Build history of the part. All positions in model axes, mm. Face numbers are marked on the shaded views. A direction names the side the tool comes from. Give positions to 0.01 mm unless a question says otherwise; leave off trailing zeros. Loops run counter-clockwise (first coordinate to the right, second up) from the corner with the lowest first, then second, coordinate; pieces in that order, holes last. Notation, with made-up numbers: M 59.5,57.25 L 64.5,57.25 A22 ccw 64.5,92.25 Z; hole C 61.5,-15.5 d8. An arc over 180 degrees is marked long. Answer as a JSON object with one key per item and string values. Group by question number.
1. Drop flat-ended pins along their axis: pin 1 Ø1.5 at (x, y) = (-16, -45.5) entering from +Z; pin 2 Ø4 at (x, z) = (-5, 3.5) entering from -Y; pin 3 Ø8 at (y, z) = (2.5, -1) entering from +X. Give the stop position or say it passes through.
2. Slice it at C-C (z = 12). List the corners of the cut face in (x, y).
3. Slice it at A-A (z = -6). List the corners of the cut face in (x, y).
4. Slice it at D-D (z = 23). List the corners of the cut face in (x, y), then the cut area to 3 significant figures.
5. 3-axis set-ups, long thin cutter, end or side, ignore diameter. For the marked faces 1, 2, 3, 4 and 5: which of +Z, -Z, +X, -X, +Y, -Y reach the whole face in a straight line?
6. Mould opens along X. For the marked faces 6, 7 and 8 say: released by +X, released by -X, zero draft, split by the parting line, or undercut.
7. Drill centre lines: line 1 along Y through (x, z) = (0, -3); line 2 along Z through (x, y) = (2.5, -22.5); line 3 along Z through (x, y) = (3, -60). Where is each one in solid material? Low to high. Write a range as [from, to].
8. Slice it at B-B (x = 0). List the corners of the cut face in (y, z), then the cut area to 3 significant figures.
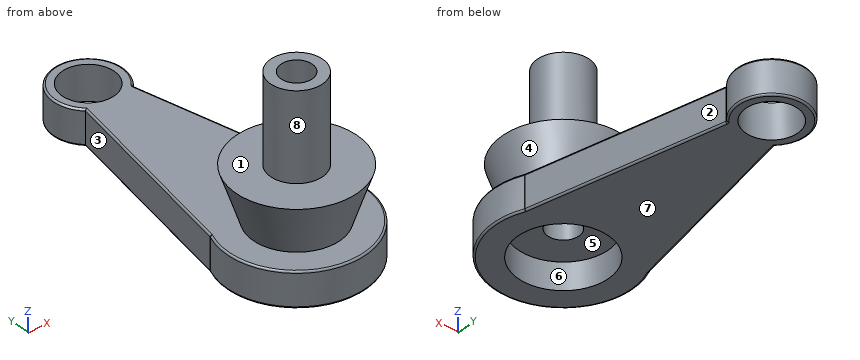
from build123d import *

# Parameters (mm, degrees)
BOSS_EXTRUDE2_DEPTH = 10
SKETCH11_R          = 7.5
CUT_EXTRUDE1_DEPTH  = 11
SKETCH12_R          = 12.5
SKETCH13_R          = 17.5
SKETCH16_R          = 7.5
BOSS_EXTRUDE3_DEPTH = 25
SKETCH17_R          = 13
CUT_EXTRUDE2_DEPTH  = 7.7
FILLET2_R           = 0.5
CUT_EXTRUDE3_REACH  = 44.3
SKETCH18_R          = 4.5


with BuildPart() as part:
    # Sketch10 → Boss-Extrude2 (new body)
    with BuildSketch(Plane.XY):
        with BuildLine():
            Line((-7, 12.658044745), (-18.304628492, -42.341955255))
            ThreePointArc((-18.304628492, -42.341955255), (0, -70.400526826), (18.304628492, -42.341955255))
            Line((18.304628492, -42.341955255), (7, 12.658044745))
            ThreePointArc((7, 12.658044745), (0, 29.799473174), (-7, 12.658044745))
        make_face()
    extrude(amount=-BOSS_EXTRUDE2_DEPTH)

    # Sketch11 → Cut-Extrude1 (cut, through all)
    with BuildSketch(Plane.XY):
        with Locations((0, 19.799473174)):
            Circle(SKETCH11_R)
    extrude(amount=-CUT_EXTRUDE1_DEPTH, mode=Mode.SUBTRACT)

    # Sketch12 → Loft1 section 0
    with BuildSketch(Plane.XY):
        with Locations((0, -50.400526826)):
            Circle(SKETCH12_R)
    # Sketch13 → Loft1 section 1
    with BuildSketch(Plane.XY.offset(15)):
        with Locations((0, -50.400526826)):
            Circle(SKETCH13_R)
    loft()

    # Sketch16 → Boss-Extrude3 (add)
    with BuildSketch(Plane.XY.offset(15)):
        with Locations((0, -50.400526826)):
            Circle(SKETCH16_R)
    extrude(amount=BOSS_EXTRUDE3_DEPTH)

    # Sketch17 → Cut-Extrude2 (cut)
    with BuildSketch(Plane(origin=(0, 0, -10), x_dir=(-1, 0, 0), z_dir=(0, 0, -1))):
        with Locations((0, -50.400526826)):
            Circle(SKETCH17_R)
    extrude(amount=-CUT_EXTRUDE2_DEPTH, mode=Mode.SUBTRACT)

    # Fillet2
    fillet2_edges = [part.edges().sort_by_distance(p)[0] for p in [
        (0, -70.400526826, -10),
        (12.652314246, -14.841955255, -10),
        (0, 29.799473174, -10),
        (12.652314246, -14.841955255, 0),
        (0, -70.400526826, 0),
        (-12.652314246, -14.841955255, 0),
        (0, 29.799473174, 0),
        (-12.652314246, -14.841955255, -10),
        (7, 12.658044745, -5),
        (18.304628492, -42.341955255, -5),
        (-18.304628492, -42.341955255, -5),
    ]]
    fillet(fillet2_edges, radius=FILLET2_R)

    # Sketch18 → Cut-Extrude3 (cut, up to next)
    with BuildSketch(Plane(origin=(0, 0, -2.3), x_dir=(-1, 0, 0), z_dir=(0, 0, -1)), mode=Mode.PRIVATE) as cut_extrude3_sk1:
        with Locations((0, -50.400526826)):
            Circle(SKETCH18_R)
    cut_extrude3_tool1 = extrude(cut_extrude3_sk1.sketch, amount=-CUT_EXTRUDE3_REACH, mode=Mode.PRIVATE) & part.part
    add(cut_extrude3_tool1.solids().sort_by_distance((0, -50.400527, -2.3))[0], mode=Mode.SUBTRACT)


solid = part.part
Established:
{
 "1": {"pin 1": "stops at z = 15", "pin 2": "stops at y = -64.08", "pin 3": "stops at x = 9.91"},
 "2": {"outline": "C 0,-50.4 d33; hole C 0,-50.4 d9"},
 "3": {"outline": "M -18.33,-42.39 A20 ccw long 18.33,-42.39 A0.5 cw 18.29,-42.29 L 7.05,12.4 A0.5 cw 7.18,12.84 A10 ccw long -7,12.66 L -18.29,-42.29 A0.5 cw Z; hole C 0,-50.4 d26; hole C 0,19.8 d15"},
 "4": {"outline": "C 0,-50.4 d15; hole C 0,-50.4 d9", "area": "113 mm^2"},
 "5": {"face 1": "+Z", "face 2": "+Z, -Z, +X", "face 3": "+Z, -Z, -X", "face 4": "none", "face 5": "-Z"},
 "6": {"face 6": "undercut", "face 7": "zero draft", "face 8": "split by the parting line"},
 "7": {"line 1": "y = [-70.4, -63.4], [-37.4, 12.3], [27.3, 29.8]", "line 2": "z = [-10, 0]", "line 3": "z = [-2.3, 15]"},
 "8": {"outline": "M -70.4,-9.5 A0.5 ccw -69.9,-10 L -63.4,-10 L -63.4,-2.3 L -54.9,-2.3 L -54.9,40 L -57.9,40 L -57.9,15 L -67.9,15 L -62.9,0 L -69.9,0 A0.5 ccw -70.4,-0.5 Z; M -45.9,-2.3 L -37.4,-2.3 L -37.4,-10 L 12.3,-10 L 12.3,0 L -37.9,0 L -32.9,15 L -42.9,15 L -42.9,40 L -45.9,40 Z; M 27.3,-10 L 29.3,-10 A0.5 ccw 29.8,-9.5 L 29.8,-0.5 A0.5 ccw 29.3,0 L 27.3,0 Z", "area": "1,100 mm^2"}
}
